Build history of the part. All positions in model axes, mm. A direction names the side the tool comes from. Round coordinates to 2 decimals unless told otherwise and drop trailing zeros. Write each loop counter-clockwise with the first axis right and the second up, starting at its lowest first coordinate (ties: lowest second). Pieces come first, ordered by that corner, then holes. Notation, with made-up numbers: M 29.5,-30 L 76.5,-30 A17 ccw 76.5,-13 Z; hole C 28,-19.75 d3. An arc over 180 degrees is marked long. Write item = value, one per line.
from build123d import *

# Parameters (mm, degrees)
CROQUIS1_R              = 3
SALIENTE_EXTRUIR1_DEPTH = 3


with BuildPart() as part:
    # Croquis1 → Saliente-Extruir1 (new body)
    with BuildSketch(Plane(origin=(0, 0, 0), x_dir=(1, 0, 0), z_dir=(0, 1, 0))):
        Polygon((0, 0), (30, 0), (30, 8.5), (33, 8.5), (33, 13.5), (33, 18.5), (30, 18.5), (30, 27), (0, 27), (0, 18.5), (-3, 18.5), (-3, 13.5), (-3, 8.5), (0, 8.5), align=None)
        with Locations(Location((15, 13.5, 0), (0, 0, 270))):
            Circle(CROQUIS1_R, mode=Mode.SUBTRACT)
    extrude(amount=SALIENTE_EXTRUIR1_DEPTH)


solid = part.part
1. Band-saw the part on A-A (z = -13.5). List the corners of the cut face in (x, y), plus the area to 3 significant figures.
Responses:
outline = M -3,0 L 12,0 L 12,3 L -3,3 Z; M 18,0 L 33,0 L 33,3 L 18,3 Z
area = 90.0 mm²
2. Mould opens along Z. For faces 4 (the face through (12.07, 1.48, -14.15)), 5 (the face through (15, 0, -17)), 6 (the face through (32, 1, -18.5)) say: pulls with the +Z half, pulls with the -Z half, needs draft (parallel to the pull), parting line crosses it, or undercut.
Responses:
face_4 = undercut
face_5 = needs draft
face_6 = pulls with the -Z half
3. Tool access for faces 1 (the face through (0, 1, -4)), 2 (the face through (-1, 1, -18.5)), 3 (the face through (31, 1, -8.5)): list every direction of +Z, -Z, +X, -X, +Y, -Y with a clear straight run to the whole face (end or side of a thin tool).
Responses:
face_1 = +Z, -X, +Y, -Y
face_2 = -Z, -X, +Y, -Y
face_3 = +Z, +X, +Y, -Y
4. Band-saw the part on C-C (y = 1.45). List the corners of the cut face in (x, z), plus the area to 3 significant figures.
Responses:
outline = M -3,-18.5 L 0,-18.5 L 0,-27 L 30,-27 L 30,-18.5 L 33,-18.5 L 33,-8.5 L 30,-8.5 L 30,0 L 0,0 L 0,-8.5 L -3,-8.5 Z; hole C 15,-13.5 d6
area = 842 mm²
5. Band-saw the part on D-D (z = -3.75). List the corners of the cut face in (x, y), plus the area to 3 significant figures.
Responses:
outline = M 0,0 L 30,0 L 30,3 L 0,3 Z
area = 90.0 mm²
6. Band-saw the part on B-B (x = 15). List the corners of the cut face in (y, z), plus the area to 3 significant figures.
Responses:
outline = M 0,-27 L 3,-27 L 3,-16.5 L 0,-16.5 Z; M 0,-10.5 L 3,-10.5 L 3,0 L 0,0 Z
area = 63.0 mm²
7. Flat gauge pins, fed straight in: pin 1 (8 mm diameter, centred on x = 27, z = -10, fed in from -Y); pin 2 (1.5 mm diameter, centred on y = 2, z = -3.5, fed in from -X); pin 3 (5.5 mm diameter, centred on x = 15, z = -13.5, fed in from -Y) (1 decimal); pin 4 (1.5 mm diameter, centred on x = -2, y = 1.5, fed in from -Z). Where does each tip first touch, or does it go through?
Responses:
pin_1 = 0
pin_2 = 0
pin_3 = through
pin_4 = -18.5
8. Probe probe 1 along X at (y, z) = (1.6, -13.5); probe 2 along X at (y, z) = (1.35, -3); probe 3 along Z at (x, y) = (12.5, 1.45). List the from-to ranges inside material, lowest first.
Responses:
probe_1 = -3 to 12, 18 to 33
probe_2 = 0 to 30
probe_3 = -27 to -15.16, -11.84 to 0
